Print and shaded views of the part. All mm, measured from the part's lowest x, y and z. A direction names the side the tool comes from. Give positions to 0.01 mm unless a question says otherwise; leave off trailing zeros. Loops run counter-clockwise (first coordinate to the right, second up) from the corner with the lowest first, then second, coordinate; pieces in that order, holes last.
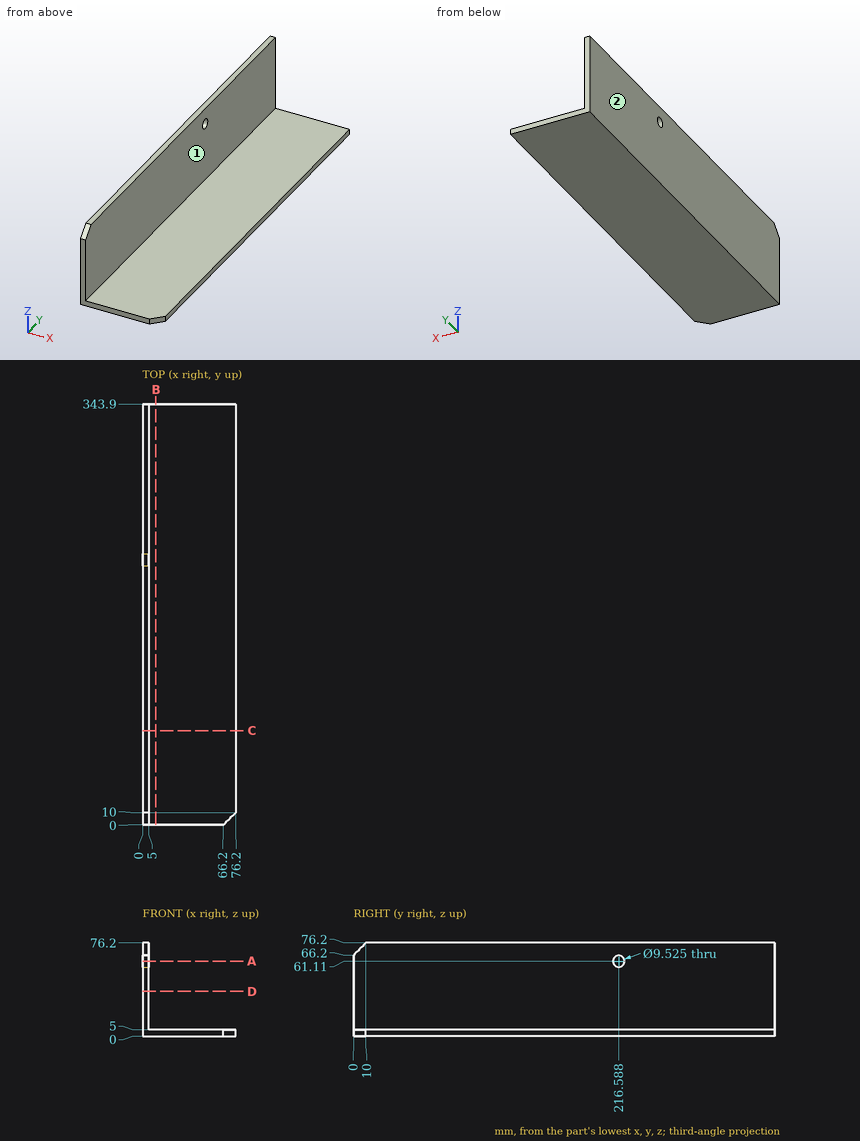
1. Saw through at D-D, the plane z = 36.5. List the corners of the cut face in (x, y).
Responses:
outline: (0, 0) - (5, 0) - (5, 343.9) - (0, 343.9) - close
2. Saw through at C-C, the plane y = 77. List the corners of the cut face in (x, z), and give its area (3 significant figures).
Responses:
outline: (0, 0) - (76.2, 0) - (76.2, 5) - (5, 5) - (5, 76.2) - (0, 76.2) - close
area: 737 mm2
3. Drop flat-ended pins along their axis: pin 1 (5 mm diameter, centred on y = 244.5, z = 46.5, fed in from +X); pin 2 (2 mm diameter, centred on x = 61, y = 216, fed in from +Z). Give the stop position or say it passes through.
Responses:
pin 1: stops at x = 5
pin 2: stops at z = 5
4. Tool access for the marked faces 1 and 2: list every direction of +Z, -Z, +X, -X, +Y, -Y with a clear straight run to the whole face (end or side of a thin tool).
Responses:
face 1: +Z, +X, +Y, -Y
face 2: +Z, -Z, -X, +Y, -Y
5. Saw through at B-B, the plane x = 11. List the corners of the cut face in (y, z).
Responses:
outline: (0, 0) - (343.9, 0) - (343.9, 5) - (0, 5) - close
6. Saw through at A-A, the plane z = 61.11. List the corners of the cut face in (x, y).
Responses:
outline: (0, 0) - (5, 0) - (5, 211.83) - (0, 211.83) - close; (0, 221.35) - (5, 221.35) - (5, 343.9) - (0, 343.9) - close
7. Probe line 1 along Y through (x, z) = (2, 61); line 2 along Z through (x, y) = (48, 324.5). List the from-to ranges inside material, lowest first.
Responses:
line 1: y = 0 to 211.83, 221.35 to 343.9
line 2: z = 0 to 5
